The listing builds one solid part. Answer for the finished solid, in the listing's coordinates (mm). Round coordinates to 2 decimals unless told otherwise and drop trailing zeros. Write each loop counter-clockwise with the first axis right and the second up, starting at its lowest first coordinate (ties: lowest second). Pieces come first, ordered by that corner, then holes. Notation, with made-up numbers: (-24.5, 66.25) - (27.5, 66.25) arc R27 ccw to (27.5, 95.25) - close; hole circle Ø11 at (33.25, 8). An arc over 180 degrees is marked (long way). Return JSON: item names as keys, results as strings. Group by question number.
(1) Find the intervals of material crossed by line 1 along Z through (x, y) = (0, -9.6); line 2 along X through (y, z) = (0, 271), in increasing order. Write a range as [from, to].
(2) This flat-tipped pin is pushed along its axis until it touches: pin 1 (3.5 mm diameter, centred on y = 0, z = 88.59, fed in from -X). Where does it stop, or does it pass through?
(3) Section A-A, the plane y = -5 is taken. Write down the section's boundary in (x, z).
(4) Section B-B, the plane z = 358.5 is taken. Write down the section's boundary in (x, y).
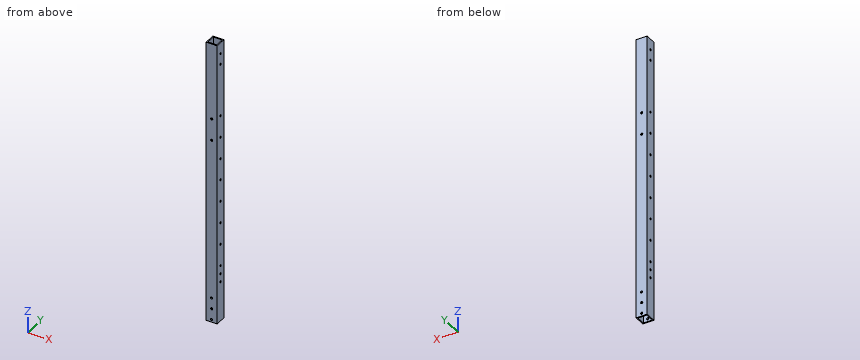
```python
from build123d import *

# Parameters (mm, degrees)
SKETCH_1_W          = 20
SKETCH_1_H          = 20
SKETCH_1_W_2        = 16
SKETCH_1_H_2        = 16
EXTRUDE_1_DEPTH     = 520
SKETCH_2_R          = 2
CUT_EXTRUDE_1_DEPTH = 521.480547187
SKETCH_3_R          = 2
CUT_EXTRUDE_2_DEPTH = 521.480547187
SKETCH_4_R          = 2
CUT_EXTRUDE_3_DEPTH = 521.480547187
SKETCH_5_R          = 2
CUT_EXTRUDE_4_DEPTH = 521.480547187


with BuildPart() as part:
    # 草图1 → 凸台-拉伸1 (new body)
    with BuildSketch(Plane.XY):
        Rectangle(SKETCH_1_W, SKETCH_1_H)
        Rectangle(SKETCH_1_W_2, SKETCH_1_H_2, mode=Mode.SUBTRACT)
    extrude(amount=EXTRUDE_1_DEPTH)

    # 草图2 → 切除-拉伸1 (cut, through all)
    with BuildSketch(Plane.XZ.offset(10)):
        with Locations((0, 5)):
            Circle(SKETCH_2_R)
        with Locations((0, 25)):
            Circle(SKETCH_2_R)
        with Locations((0, 45)):
            Circle(SKETCH_2_R)
    extrude(amount=-CUT_EXTRUDE_1_DEPTH, mode=Mode.SUBTRACT)

    # 草图3 → 切除-拉伸2 (cut, through all)
    with BuildSketch(Plane(origin=(10, 0, 0), x_dir=(0, 0, -1), z_dir=(1, 0, 0))):
        with Locations(Location((-500, 0, 0), (0, 0, 90))):
            Circle(SKETCH_3_R)
        with Locations(Location((-480, 0, 0), (0, 0, 90))):
            Circle(SKETCH_3_R)
    extrude(amount=-CUT_EXTRUDE_2_DEPTH, mode=Mode.SUBTRACT)

    # 草图4 → 切除-拉伸3 (cut, through all)
    with BuildSketch(Plane(origin=(10, 0, 0), x_dir=(0, 0, -1), z_dir=(1, 0, 0))):
        with Locations(Location((-103.589838486, 0, 0), (0, 0, 90))):
            Circle(SKETCH_4_R)
        with Locations(Location((-88.589838486, 0, 0), (0, 0, 90))):
            Circle(SKETCH_4_R)
        with Locations(Location((-73.589838486, 0, 0), (0, 0, 90))):
            Circle(SKETCH_4_R)
        with Locations(Location((-143.589838486, 0, 0), (0, 0, 90))):
            Circle(SKETCH_4_R)
        with Locations(Location((-183.589838486, 0, 0), (0, 0, 90))):
            Circle(SKETCH_4_R)
        with Locations(Location((-223.589838486, 0, 0), (0, 0, 90))):
            Circle(SKETCH_4_R)
        with Locations(Location((-263.589838486, 0, 0), (0, 0, 90))):
            Circle(SKETCH_4_R)
        with Locations(Location((-303.589838486, 0, 0), (0, 0, 90))):
            Circle(SKETCH_4_R)
        with Locations(Location((-343.589838486, 0, 0), (0, 0, 90))):
            Circle(SKETCH_4_R)
        with Locations(Location((-383.589838486, 0, 0), (0, 0, 90))):
            Circle(SKETCH_4_R)
    extrude(amount=-CUT_EXTRUDE_3_DEPTH, mode=Mode.SUBTRACT)

    # 草图5 → 切除-拉伸4 (cut, through all)
    with BuildSketch(Plane.XZ.offset(10)):
        with Locations((0, 380)):
            Circle(SKETCH_5_R)
        with Locations((0, 340)):
            Circle(SKETCH_5_R)
    extrude(amount=-CUT_EXTRUDE_4_DEPTH, mode=Mode.SUBTRACT)


solid = part.part
```
Working result:
{
 "1": {"line 1": "z = [0, 3], [7, 23], [27, 43], [47, 338], [342, 378], [382, 520]", "line 2": "x = [-10, -8], [8, 10]"},
 "2": {"pin 1": "passes through"},
 "3": {"outline": "(-10, 0) - (-8, 0) - (-8, 520) - (-10, 520) - close; (8, 0) - (10, 0) - (10, 520) - (8, 520) - close"},
 "4": {"outline": "(-10, -10) - (10, -10) - (10, 10) - (-10, 10) - close; hole (-8, -8) - (8, -8) - (8, 8) - (-8, 8) - close"}
}
